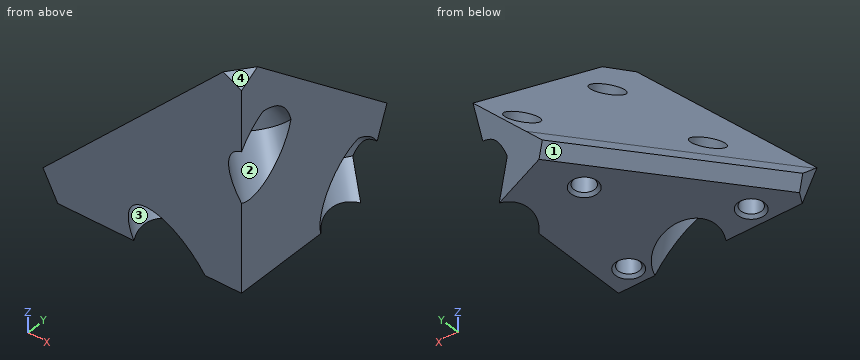
```python
from build123d import *

# Parameters (mm, degrees)
BOSS_EXTRUDE1_DEPTH                            = 14
CUT_EXTRUDE1_DEPTH                             = 18.804493815
CUT_EXTRUDE1_DEPTH_BACK                        = 18.804493815
BOSS_EXTRUDE2_DEPTH                            = 2
CSK_FOR_M2_FLAT_HEAD_MACHINE_SCREW1_AT_2_COUNT = 2
CSK_FOR_M2_FLAT_HEAD_MACHINE_SCREW1_AT_2_PITCH = 11.412712211
CSK_FOR_M2_FLAT_HEAD_MACHINE_SCREW1_AT_3_COUNT = 2
CSK_FOR_M2_FLAT_HEAD_MACHINE_SCREW1_AT_3_PITCH = 11
M2X0_4_TAPPED_HOLE1_D                          = 1.6
M2X0_4_TAPPED_HOLE1_DEPTH                      = 3.5
M2X0_4_TAPPED_HOLE1_CSINK_D                    = 2.05
M2X0_4_TAPPED_HOLE1_CSINK_ANGLE                = 90
M2X0_4_TAPPED_HOLE1_TIP                        = 0.480688495
BOSS_EXTRUDE5_REACH                            = 20.765
SKETCH12_W                                     = 1.58113883
SKETCH12_H                                     = 18.073922282
CUT_EXTRUDE3_DEPTH                             = 20.541337939
CUT_EXTRUDE3_DEPTH_BACK                        = 20.541337939


with BuildPart() as part:
    # Sketch1 → Boss-Extrude1 (new body)
    with BuildSketch(Plane(origin=(0, 0, 0), x_dir=(1, 0, 0), z_dir=(0, 1, 0))):
        Polygon((-7.778174593, 7.778174593), (7.778174593, -7.778174593), (7.778174593, 7.778174593), align=None)
    extrude(amount=BOSS_EXTRUDE1_DEPTH)

    # Sketch2 → Cut-Extrude1 (cut, two sides: drawn at the far end of the back side and taken through both)
    with BuildSketch(Plane(origin=(0, 0, 0), x_dir=(0, -1, 0), z_dir=(-0.7071067811865476, 0, -0.7071067811865476)).offset(-CUT_EXTRUDE1_DEPTH_BACK)):
        Polygon((0, 0), (-14, -8.082903769), (-14, 0), align=None)
    extrude(amount=CUT_EXTRUDE1_DEPTH + CUT_EXTRUDE1_DEPTH_BACK, mode=Mode.SUBTRACT)

    # Sketch7 → Boss-Extrude2 (add)
    with BuildSketch(Plane(origin=(0, 0, -7.778174593), x_dir=(-1, 0, 0), z_dir=(0, 0, -1))):
        Polygon((-7.778174593, 0), (7.778174593, 0), (-3.65277754, 14), (-7.778174593, 14), align=None)
    extrude(amount=BOSS_EXTRUDE2_DEPTH)

    # Sketch4 → CSK for M2 Flat Head Machine Screw1 (revolve, cut)
    with BuildSketch(Plane(origin=(12.828546783, -2.102885683, -5.050372189), x_dir=(-0.048813033433799426, 0.7492053416010188, -0.6605366332638121), z_dir=(0.7890610165044198, 0.4343861831556179, 0.43438618315561783))):
        Polygon((0, 0), (0, 13.921032743), (1.2, 13.2), (1.2, 11), (2.2, 10), (2.2, 0), align=None)
    csk_for_m2_flat_head_machine_screw1 = revolve(axis=Axis((16.717111749, -5.277885683, -8.938937156), (-0.6123724356957967, 0.4999999999999948, 0.6123724356957967)), mode=Mode.SUBTRACT)

    # CSK for M2 Flat Head Machine Screw1 at 2: CSK for M2 Flat Head Machine Screw1 ×2
    with Locations(*[Vector(-0.030978910540443338, 0.7588252361140443, -0.6505571213492264) * (i * CSK_FOR_M2_FLAT_HEAD_MACHINE_SCREW1_AT_2_PITCH) for i in range(1, CSK_FOR_M2_FLAT_HEAD_MACHINE_SCREW1_AT_2_COUNT)]):
        add(csk_for_m2_flat_head_machine_screw1, mode=Mode.SUBTRACT)

    # CSK for M2 Flat Head Machine Screw1 at 3: CSK for M2 Flat Head Machine Screw1 ×2
    with Locations(*[Vector(-0.7071067811865477, 0, -0.7071067811865474) * (i * CSK_FOR_M2_FLAT_HEAD_MACHINE_SCREW1_AT_3_PITCH) for i in range(1, CSK_FOR_M2_FLAT_HEAD_MACHINE_SCREW1_AT_3_COUNT)]):
        add(csk_for_m2_flat_head_machine_screw1, mode=Mode.SUBTRACT)

    # M2x0.4 Tapped Hole1
    with Locations(Plane(origin=(0, 0, -9.778174593), x_dir=(-1, 0, 0), z_dir=(0, 0, -1))):
        with Locations((-2.778174593, 9.5), (-5.778174593, 1.5), (3.721825407, 1.5)):
            CounterSinkHole(M2X0_4_TAPPED_HOLE1_D / 2, M2X0_4_TAPPED_HOLE1_CSINK_D / 2, depth=M2X0_4_TAPPED_HOLE1_DEPTH, counter_sink_angle=M2X0_4_TAPPED_HOLE1_CSINK_ANGLE)
            with Locations((0, 0, -(M2X0_4_TAPPED_HOLE1_DEPTH + M2X0_4_TAPPED_HOLE1_TIP / 2))):  # 118° drill point
                Cone(0, M2X0_4_TAPPED_HOLE1_D / 2, M2X0_4_TAPPED_HOLE1_TIP, mode=Mode.SUBTRACT)

    # Boss-Extrude5: up to this face of the body (flat: up to its plane)
    boss_extrude5_end = Plane(part.part.faces().sort_by_distance((-2.062698527, 7, -8.778174593))[0])
    # Sketch12 → Boss-Extrude5 (add, up to the picked face)
    with BuildSketch(Plane(origin=(0, 0, 0), x_dir=(0.4743416490252608, -0.3872983346207397, 0.7905694150420935), z_dir=(-0.6123724356957969, 0.4999999999999949, 0.6123724356957962)), mode=Mode.PRIVATE) as boss_extrude5_sk1:
        with Locations((-10.629268516, 4.117611591)):
            Rectangle(SKETCH12_W, SKETCH12_H)
    boss_extrude5_tool1 = split(extrude(boss_extrude5_sk1.sketch, amount=-BOSS_EXTRUDE5_REACH, mode=Mode.PRIVATE), bisect_by=boss_extrude5_end, keep=Keep.BOTH, mode=Mode.PRIVATE)
    add(boss_extrude5_tool1.solids().sort_by(Axis((-2.437699, 7.306186, -8.403175), (0.6123724356957969, -0.4999999999999949, -0.6123724356957962)))[0])

    # Sketch9 → Cut-Extrude3 (cut, two sides: drawn at the far end of the back side and taken through both)
    with BuildSketch(Plane(origin=(0, 0, 0), x_dir=(0.4743416490252609, -0.3872983346207397, 0.7905694150420934), z_dir=(-0.6123724356957968, 0.49999999999999495, 0.6123724356957964)).offset(-CUT_EXTRUDE3_DEPTH_BACK)):
        Polygon((8.238699101, 6.11934955), (8.049844719, 4.024922359), (9.838699101, 4.91934955), align=None)
        Polygon((-9.630983549, -4.815491775), (-11.419837931, -5.709918966), (-11.419837931, -3.709918966), align=None)
        Polygon((-4.620438725, 15.76370292), (-11.419837931, 12.364003317), (-11.419837931, 20.863252325), align=None)
    extrude(amount=CUT_EXTRUDE3_DEPTH + CUT_EXTRUDE3_DEPTH_BACK, mode=Mode.SUBTRACT)


solid = part.part
```
Build history of the part. All positions in model axes, mm. Face numbers are marked on the shaded views. Coordinates: 2 decimals unless noted, no trailing zeros. Write each loop counter-clockwise with the first axis right and the second up, starting at its lowest first coordinate (ties: lowest second). Pieces come first, ordered by that corner, then holes.
1. Pull direction X, two halves, no side cores. Call the marked faces 1, 2, 3 and 4: released by +X, released by -X, zero draft, split by the parting line, or undercut.
Answer block:
face 1: released by -X
face 2: undercut
face 3: undercut
face 4: released by +X
2. Drill centre lines: probe 1 along X at (y, z) = (1.5, -8.75); probe 2 along X at (y, z) = (1.5, -7.55); probe 3 along X at (y, z) = (9.5, -6.25). Where is each one in solid material? Low to high.
Answer block:
probe 1: x = -7.53 to -4.52, -2.92 to -1.93, 3.61 to 4.98, 6.58 to 7.78
probe 2: x = -6.33 to -4.52, -2.92 to -2.58, 2.81 to 4.98, 6.58 to 7.78
probe 3: x = 1.51 to 2.03, 3.53 to 5.47
3. Band-saw the part on A-A, the plane y = 5.75. Give the cut face in (x, z).
Answer block:
outline: (-4.33, -9.03) - (-3.08, -9.78) - (7.78, -9.78) - (7.78, 3.08) - close
4. Band-saw the part on B-B, the plane z = 5. Give the cut face in (x, y).
Answer block:
outline: (5, 0) - (7.78, 0) - (7.78, 3.4) - close
5. Drop flat-ended pins along their axis: pin 1 (2.5 mm diameter, centred on x = 2.78, y = 9.5, fed in from -Z); pin 2 (1 mm diameter, centred on x = -3.72, y = 1.5, fed in from -Z); pin 3 (1.5 mm diameter, centred on x = 1.5, y = 4.5, fed in from +Z); pin 4 (1.8 mm diameter, centred on x = 5.78, y = 1.5, fed in from -Z) (3 decimals). Give the stop position or say it passes through.
Answer block:
pin 1: stops at z = -9.78
pin 2: stops at z = -6.1
pin 3: stops at z = -1.21
pin 4: stops at z = -9.655
